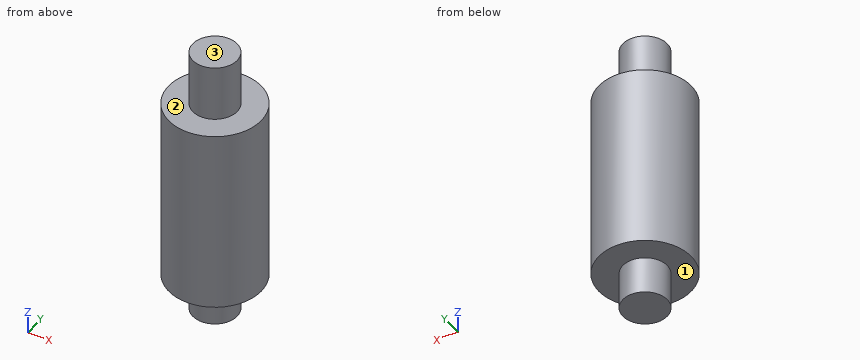
Autodesk Inventor part; units mm, degrees
ref_plane "YZ Plane" through (0, 0, 0) normal (1, 0, 0) x (0, 1, 0)
ref_plane "XZ Plane" through (0, 0, 0) normal (0, 1, 0) x (-1, 0, 0)
ref_plane "XY Plane" through (0, 0, 0) normal (0, 0, 1) x (1, 0, 0)
sketch "Sketch1" plane through (0, 0, 0) normal (0, 0, 1) x (1, 0, 0)
  circle A0 centre (-2.0967, 1.4241) radius 1.2
  point P0 (0, 0)
  dimension "d0" = 2.4
extrude "Extrusion1" add sketch "Sketch1" along normal blind 15
ref_plane "Work Plane1" through (-2.0967, 1.4241, 12) normal (0, 0, 1) x (1, 0, 0)
sketch "Sketch3" plane through (-2.0967, 1.4241, 12) normal (0, 0, 1) x (1, 0, 0)
  circle A0 centre (0, 0) radius 1.2
  circle A1 centre (0, 0) radius 1.2
  circle A2 centre (0, 0) radius 2.5
  point P0 (2.0967, -1.4241)
  dimension "d4" = 5
extrude "Extrusion2" add sketch "Sketch3" against normal blind 10
properties part number "M2" material "Silver"
Model file for the job. Use its own axes, mm. Face numbers are marked on the shaded views. A direction names the side the tool comes from. Coordinates: 2 decimals unless noted, no trailing zeros. Order: outer loops, then holes, each group sorted by start corner. A loop starts at its lowest first (then second) coordinate and runs counter-clockwise, first axis right, second up. Notation, with made-up numbers: M -31,19 L 17,19 A14 cw 17,33 Z; hole C 73.25,-9.75 d5. An arc over 180 degrees is marked long. Answer as CSV lines item,"result".
(1) Band-saw the part on C-C, the plane z = 10. List the corners of the cut face in (x, y).
Geometry says:
outline,"C -2.1,1.42 d5"
(2) Flat gauge pins, fed straight in: pin 1 (1 mm diameter, centred on y = 3, z = 12, fed in from +X); pin 2 (2 mm diameter, centred on y = 0, z = 7, fed in from -X). Where does each tip first touch, or does it go through?
Geometry says:
pin 1,"stops at x = 0.16"
pin 2,"stops at x = -4.56"
(3) Wall check: line 1 along Z through (x, y) = (-1.6, 2.9); line 2 along Y through (x, z) = (-2.1, 1); line 3 along Y through (x, z) = (-3.4, 7.25). Give the ranges that are in metal, low to high.
Geometry says:
line 1,"z = 2 to 12"
line 2,"y = 0.22 to 2.62"
line 3,"y = -0.71 to 3.56"
(4) 3-axis set-ups, long thin cutter, end or side, ignore diameter. For the marked faces 1, 2 and 3: which of +Z, -Z, +X, -X, +Y, -Y reach the whole face in a straight line?
Geometry says:
face 1,"-Z"
face 2,"+Z"
face 3,"+Z, +X, -X, +Y, -Y"
(5) Band-saw the part on D-D, the plane x = -3.95. List the corners of the cut face in (y, z).
Geometry says:
outline,"M -0.25,2 L 3.1,2 L 3.1,12 L -0.25,12 Z"
(6) Band-saw the part on A-A, the plane x = -1.8. List the corners of the cut face in (y, z), then the cut area to 3 significant figures.
Geometry says:
outline,"M -1.06,2 L 0.26,2 L 0.26,0 L 2.59,0 L 2.59,2 L 3.91,2 L 3.91,12 L 2.59,12 L 2.59,15 L 0.26,15 L 0.26,12 L -1.06,12 Z"
area,"61.3 mm2"
(7) Band-saw the part on B-B, the plane y = 0.6. List the corners of the cut face in (x, z), then the cut area to 3 significant figures.
Geometry says:
outline,"M -4.46,2 L -2.97,2 L -2.97,0 L -1.22,0 L -1.22,2 L 0.26,2 L 0.26,12 L -1.22,12 L -1.22,15 L -2.97,15 L -2.97,12 L -4.46,12 Z"
area,"55.9 mm2"
